Autodesk Fusion 360 part; units mm, degrees
sketch "extrusion" plane through (0, 0, 0) normal (0, 1, 0) x (1, 0, 0)
  line L0 (-82.5, -8) -> (-62.5, -8)
  line L1 (-62.5, -8) -> (-62.5, 0)
  line L2 (-62.5, 0) -> (62.5, 0)
  line L3 (62.5, 0) -> (62.5, -8)
  line L4 (62.5, -8) -> (82.5, -8)
  line L5 (-60.5, -12) -> (-60.5, -2)
  line L6 (-60.5, -2) -> (60.5, -2)
  line L7 (60.5, -2) -> (60.5, -12)
  line L8 (-82.5, -12) -> (-60.5, -12)
  line L9 (60.5, -12) -> (82.5, -12)
  line L10 (-82.5, -8) -> (-82.5, -12)
  line L11 (82.5, -8) -> (82.5, -12)
  dimension "d1" = 125
  dimension "d2" = 8
  dimension "d3" = 20
  dimension "d4" = 8
  dimension "d5" = 20
extrude "Extrude1" add sketch "extrusion" along normal mid plane 140
sketch "top holes" plane through (0, 0, 12) normal (0, 0, 1) x (-1, 0, 0)
  circle A0 centre (71.5, -53.75) radius 3
  line L0 (82.5, -70) -> (60.5, -70)
  dimension "d11" = 6
  dimension "d12" = 16.25
extrude "Extrude2" cut sketch "top holes" against normal blind 4
mirror "Mirror1" about plane through (0, 0, 0) normal (1, 0, 0) of "Extrude2"
mirror "Mirror2" about plane through (0, 0, 0) normal (0, 1, 0) of "Extrude2", "Mirror1"
Check sheet for the modelled part. Datum: model origin and axes. Units: mm. A direction names the side the tool comes from. Round coordinates to 2 decimals unless told otherwise and drop trailing zeros. Order: outer loops, then holes, each group sorted by start corner. A loop starts at its lowest first (then second) coordinate and runs counter-clockwise, first axis right, second up. Notation, with made-up numbers: M 53,-9.75 L 95,-9.75 A21 cw 95,16.25 Z; hole C 66,2 d4. An arc over 180 degrees is marked long. One line per item, written item: value. Start each with the question number.
1. Scan lines: line 1 along Y through (x, z) = (71.5, 10.4); line 2 along X through (y, z) = (-27.5, 8.25); line 3 along X through (y, z) = (-8, 5.5). Record each from-to range of solid material in increasing order.
2. Section check B-B on z = 5.75. Enter the section's corners in (x, y), and give its area (3 significant figures).
3. Access from +Z, -Z, +X, -X, +Y, -Y to the whole of each face (thin tool, end or side, straight path). Record for faces 1 (the flat face through (72, -1, 8)), 2 (the flat face through (-60.5, -1, 7)), 3 (the flat face through (71, -1, 12)), 4 (the flat face through (-73, -1, 8)).
4. Section check C-C on x = -71.5. Enter the section's corners in (y, z), and give its area (3 significant figures).
5. Release check for a two-part mould opening along Y. For faces 5 (the flat face through (62.5, -1, 4)), 6 (the flat face through (0, -70, 1)), 7 (the cylindrical face through (71.109, 56.724, 10.028)) record: released by +Y, released by -Y, zero draft, split by the parting line, or undercut.
6. Section check A-A on y = 53.75. Enter the section's corners in (x, z).
7. Section check D-D on y = -3. Enter the section's corners in (x, z).
8. Gauge pin test, flat ends, axial feed: P1, Ø9.5, axis at x = 71.5, y = 53.75, coming from the -Z side; P2, Ø4, axis at y = 0.5, z = 2.5, coming from the +X side; P3, Ø10, axis at x = -49.5, y = -39, coming from the +Z side. Record the tip position at first contact, or that the pin passes through.
Results found:
1. line 1: -70 to -56.75, -50.75 to 50.75, 56.75 to 70
1. line 2: -82.5 to -60.5, 60.5 to 82.5
1. line 3: -62.5 to -60.5, 60.5 to 62.5
2. outline: M -62.5,-70 L -60.5,-70 L -60.5,70 L -62.5,70 Z; M 60.5,-70 L 62.5,-70 L 62.5,70 L 60.5,70 Z
2. area: 560 mm^2
3. face 1: -Z, +X, +Y, -Y
3. face 2: +Z, +Y, -Y
3. face 3: +Z, +X, -X, +Y, -Y
3. face 4: -Z, -X, +Y, -Y
4. outline: M -70,8 L -56.75,8 L -56.75,12 L -70,12 Z; M -50.75,8 L 50.75,8 L 50.75,12 L -50.75,12 Z; M 56.75,8 L 70,8 L 70,12 L 56.75,12 Z
4. area: 512 mm^2
5. face 5: zero draft
5. face 6: released by -Y
5. face 7: undercut
6. outline: M -82.5,8 L -74.5,8 L -74.5,12 L -82.5,12 Z; M -68.5,8 L -62.5,8 L -62.5,0 L 62.5,0 L 62.5,8 L 68.5,8 L 68.5,12 L 60.5,12 L 60.5,2 L -60.5,2 L -60.5,12 L -68.5,12 Z; M 74.5,8 L 82.5,8 L 82.5,12 L 74.5,12 Z
7. outline: M -82.5,8 L -62.5,8 L -62.5,0 L 62.5,0 L 62.5,8 L 82.5,8 L 82.5,12 L 60.5,12 L 60.5,2 L -60.5,2 L -60.5,12 L -82.5,12 Z
8. P1: z = 8
8. P2: x = 62.5
8. P3: z = 2
